from build123d import *

# Parameters (mm, degrees)
BOSS_EXTRUDE1_DEPTH = 2
SKETCH2_R           = 1.55
CUT_EXTRUDE1_DEPTH  = 2
CHAMFER1_SIZE       = 0.1


with BuildPart() as part:
    # Sketch1 → Boss-Extrude1 (new body)
    with BuildSketch(Plane.XY):
        with BuildLine():
            Line((-12, 2.5), (12, 2.5))
            ThreePointArc((12, 2.5), (14.5, 0), (12, -2.5))
            Line((12, -2.5), (-12, -2.5))
            ThreePointArc((-12, -2.5), (-14.5, 0), (-12, 2.5))
        make_face()
    extrude(amount=BOSS_EXTRUDE1_DEPTH)

    # Sketch2 → Cut-Extrude1 (cut)
    with BuildSketch(Plane.XY.offset(2)):
        with Locations((-12, 0)):
            Circle(SKETCH2_R)
        with Locations((12, 0)):
            Circle(SKETCH2_R)
    extrude(amount=-CUT_EXTRUDE1_DEPTH, mode=Mode.SUBTRACT)

    # Chamfer1
    chamfer1_edges = [part.edges().sort_by_distance(p)[0] for p in [
        (14.5, 0, 2),
        (0, 2.5, 2),
        (-13.55, 0, 0),
        (-13.55, 0, 2),
        (10.45, 0, 0),
        (10.45, 0, 2),
        (-14.5, 0, 2),
        (0, 2.5, 0),
        (14.5, 0, 0),
        (0, -2.5, 0),
        (-14.5, 0, 0),
        (0, -2.5, 2),
    ]]
    chamfer(chamfer1_edges, length=CHAMFER1_SIZE)


solid = part.part
Work out the finished part from the listing and answer in its coordinate system (mm). Give positions to 0.01 mm unless a question says otherwise; leave off trailing zeros. Loops run counter-clockwise (first coordinate to the right, second up) from the corner with the lowest first, then second, coordinate; pieces in that order, holes last. Notation, with made-up numbers: (-25, 1.25) - (5, 1.25) arc R25 cw to (5, 17.25) - close; hole circle Ø1 at (12.5, -10.75). An arc over 180 degrees is marked (long way). Answer in a Markdown table with one row per item. Add a question column.
Q1. Determine the mould class of faces 1 (the flat face through (0, 0, 2)), 2 (the cylindrical face through (-13.23, -0.94, 1.01)), 3 (the cylindrical face through (-14.5, -0.1, 1)) for opening direction X: released by +X, released by -X, zero draft, split by the parting line, or undercut.
Q2. The part is cut by section A-A (y = 0). Determine the outline of the cut face in (x, z), and give its area (3 significant figures).
Q3. Consider line 1 along Y through (x, z) = (12, 0.5); line 2 along X through (y, z) = (1, 1.1); line 3 along X through (y, z) = (0.5, 0.9). Determine where each line is inside the solid, lowest interval first.
Q4. The part is cut by section B-B (z = 0.8). Determine the outline of the cut face in (x, y), and give its area (3 significant figures).
Solution:
| question | item | result |
|---|---|---|
| 1 | face 1 | zero draft |
| 1 | face 2 | undercut |
| 1 | face 3 | released by -X |
| 2 | outline | (-14.5, 0.1) - (-14.4, 0) - (-13.65, 0) - (-13.55, 0.1) - (-13.55, 1.9) - (-13.65, 2) - (-14.4, 2) - (-14.5, 1.9) - close; (-10.45, 0.1) - (-10.35, 0) - (10.35, 0) - (10.45, 0.1) - (10.45, 1.9) - (10.35, 2) - (-10.35, 2) - (-10.45, 1.9) - close; (13.55, 0.1) - (13.65, 0) - (14.4, 0) - (14.5, 0.1) - (14.5, 1.9) - (14.4, 2) - (13.65, 2) - (13.55, 1.9) - close |
| 2 | area | 45.5 mm² |
| 3 | line 1 | y = -2.5 to -1.55, 1.55 to 2.5 |
| 3 | line 2 | x = -14.29 to -13.18, -10.82 to 10.82, 13.18 to 14.29 |
| 3 | line 3 | x = -14.45 to -13.47, -10.53 to 10.53, 13.47 to 14.45 |
| 4 | outline | (-12, -2.5) - (12, -2.5) arc R2.5 ccw to (12, 2.5) - (-12, 2.5) arc R2.5 ccw to start; hole circle Ø3.1 at (-12, 0); hole circle Ø3.1 at (12, 0) |
| 4 | area | 125 mm² |
